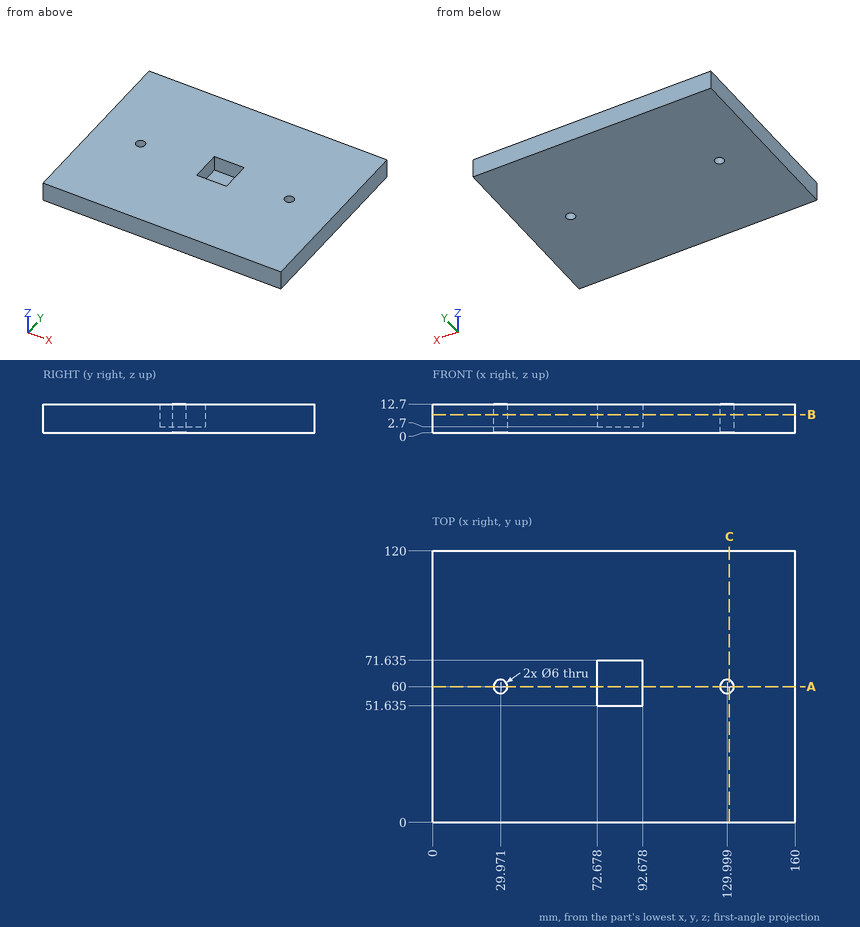
Input: dimensioned drawing with shaded views. Units: mm. Origin: part minimum x, y, z. Coordinates: 2 decimals unless noted, no trailing zeros. Write each loop counter-clockwise with the first axis right and the second up, starting at its lowest first coordinate (ties: lowest second). Pieces come first, ordered by that corner, then holes. Notation, with made-up numbers: M 51.5,5.25 L 104.5,5.25 A33 ccw 104.5,42.25 Z; hole C 19,2.25 d1. An arc over 180 degrees is marked long. Use a Markdown table: item, result.
1) Section C-C, the plane x = 131. Output: boundary loops of the cut face in (y, z), then the cut area to 3 significant figures.
Conclusion:
| item | result |
|---|---|
| outline | M 0,0 L 57.17,0 L 57.17,12.7 L 0,12.7 Z; M 62.83,0 L 120,0 L 120,12.7 L 62.83,12.7 Z |
| area | 1,450 mm^2 |
2) Ray query, L1, parallel to X at y = 60, z = 9.75; L2, parallel to X at y = 54.5, z = 12. Return the intervals inside material, ascending.
Conclusion:
| item | result |
|---|---|
| L1 | x = 0 to 26.97, 32.97 to 72.68, 92.68 to 127, 133 to 160 |
| L2 | x = 0 to 72.68, 92.68 to 160 |
3) Section B-B, the plane z = 8. Output: boundary loops of the cut face in (x, y) (1 decimal), then the cut area to 3 significant figures.
Conclusion:
| item | result |
|---|---|
| outline | M 0,0 L 160,0 L 160,120 L 0,120 Z; hole C 30,60 d6; hole M 72.7,51.6 L 92.7,51.6 L 92.7,71.6 L 72.7,71.6 Z; hole C 130,60 d6 |
| area | 18,700 mm^2 |
4) Section A-A, the plane y = 60. Output: boundary loops of the cut face in (x, z).
Conclusion:
| item | result |
|---|---|
| outline | M 0,0 L 26.97,0 L 26.97,12.7 L 0,12.7 Z; M 32.97,0 L 127,0 L 127,12.7 L 92.68,12.7 L 92.68,2.7 L 72.68,2.7 L 72.68,12.7 L 32.97,12.7 Z; M 133,0 L 160,0 L 160,12.7 L 133,12.7 Z |
